```python
from build123d import *

# Parameters (mm, degrees)
F1_DEPTH = 14
F3_DEPTH = 23.7
F4_R     = 2


with BuildPart() as f1:
    # F0 (on Front) → F1 (new body)
    with BuildSketch(Plane.XZ):
        with BuildLine():
            ThreePointArc((27, -8.005587), (26.611392, -6.072957), (25.505976, -4.440741))
            ThreePointArc((25.505976, -4.440741), (13.780093, 3.288774), (0, 6))
            ThreePointArc((0, 6), (-13.780093, 3.288774), (-25.505976, -4.440741))
            ThreePointArc((-25.505976, -4.440741), (-26.611392, -6.072957), (-27, -8.005587))
            Line((-27, -8.005587), (-27, -21))
            ThreePointArc((-27, -21), (-24.071068, -28.071068), (-17, -31))
            Line((-17, -31), (17, -31))
            ThreePointArc((17, -31), (24.071068, -28.071068), (27, -21))
            Line((27, -21), (27, -8.005587))
        make_face()
        with BuildLine():
            ThreePointArc((-22, -8.005587), (0, 1), (22, -8.005587))
            Line((22, -8.005587), (22, -21))
            ThreePointArc((22, -21), (20.535534, -24.535534), (17, -26))
            Line((17, -26), (-17, -26))
            ThreePointArc((-17, -26), (-20.535534, -24.535534), (-22, -21))
            Line((-22, -21), (-22, -8.005587))
        make_face(mode=Mode.SUBTRACT)
    extrude(amount=F1_DEPTH)

    # F2 (on Top) → F3 (cut)
    with BuildSketch(Plane.XY):
        with BuildLine():
            ThreePointArc((0, -8.25), (0.883883, -7.883883), (1.25, -7))
            ThreePointArc((1.25, -7), (0.883883, -6.116117), (0, -5.75))
            Line((0, -5.75), (0, -8.25))
        make_face()
        with BuildLine():
            Line((0, -8.25), (0, -5.75))
            ThreePointArc((0, -5.75), (-1.25, -7), (0, -8.25))
        make_face()
    extrude(amount=F3_DEPTH, mode=Mode.SUBTRACT)

    # F4
    f4_edges = [f1.edges().sort_by_distance(p)[0] for p in [
        (0, -14, 1),
        (22, -14, -14.502794),
        (20.535534, -14, -24.535534),
        (0, 0, -26),
        (0, 0, 1),
        (0, 0, -31),
        (0, -14, -31),
    ]]
    fillet(f4_edges, radius=F4_R)


solid = f1.part
```
CAD build for the part. Positions are in the model's coordinates, mm. A direction names the side the tool comes from. Round coordinates to 2 decimals unless told otherwise and drop trailing zeros. Loops run counter-clockwise (first coordinate to the right, second up) from the corner with the lowest first, then second, coordinate; pieces in that order, holes last. Notation, with made-up numbers: M 83.25,40 L 91.25,40 A22 cw 91.25,72 Z; hole C 52,-17 d10. An arc over 180 degrees is marked long. Use a Markdown table: item, result. Add a question column.
(1) Cut at A-A (z = -19). Give the cut face in (x, y), and give its area (3 significant figures).
(2) Which spindle directions (+Z, -Z, +X, -X, +Y, -Y) get a long thin tool onto all of the face, cutting with end or side? Do faces 1 (the face through (-0.24, -0.57, -26.6)), 2 (the face through (-22.6, -13.43, -13.99)), 3 (the face through (0, -5, 1)), 4 (the face through (-27, -7, -14)), 5 (the face through (-24.15, -6.93, -27.99)). Say none if no direction does.
(3) Pull direction X, two halves, no side cores. Call faces 6 (the face through (-26.4, -13.43, -14.59)), 7 (the face through (22.6, -0.57, -14.19)), 8 (the face through (-3.8, 0, -28.3)): +X half, -X half, draft (parallel to the pull), parting line (faces both ways), or undercut.
(4) Cut at B-B (y = -3.75). Give the cut face in (x, z) (3 decimals), and give its area (3 significant figures).
(5) Cut at C-C (y = -1). Give the cut face in (x, z) (3 decimals), and give its area (3 significant figures).
(6) Drill centre lines: line 1 (X direction, y = -2.5, z = -13); line 2 (Z direction, x = -1, y = -5.25); line 3 (Z direction, x = 20, y = -0.5). Where is each one in solid material? Low to high.
(7) Flat gauge pins, fed straight in: pin 1 (1 mm diameter, centred on y = -7, z = -25, fed in from -X); pin 2 (1.5 mm diameter, centred on x = 13, y = -4, fed in from +Z); pin 3 (10 mm diameter, centred on x = 8, z = -18.5, fed in from -Y); pin 4 (2 mm diameter, centred on x = 6, y = -3, fed in from +Z). Where does each tip first touch, or does it go through?
Geometry says:
| question | item | result |
|---|---|---|
| 1 | outline | M -27,-12 A2 ccw -25,-14 L -24,-14 A2 ccw -22,-12 L -22,-2 A2 ccw -24,0 L -25,0 A2 ccw -27,-2 Z; M 22,-12 A2 ccw 24,-14 L 25,-14 A2 ccw 27,-12 L 27,-2 A2 ccw 25,0 L 24,0 A2 ccw 22,-2 Z |
| 1 | area | 133 mm² |
| 2 | face 1 | +Y |
| 2 | face 2 | -Y |
| 2 | face 3 | +Y, -Y |
| 2 | face 4 | +Z, -Z, -X, +Y, -Y |
| 2 | face 5 | -Z, -X, +Y, -Y |
| 3 | face 6 | -X half |
| 3 | face 7 | undercut |
| 3 | face 8 | draft |
| 4 | outline | M -27,-21 A10 ccw -17,-31 L 17,-31 A10 ccw 27,-21 L 27,-8.006 A5 ccw 25.506,-4.441 A36.375 ccw 0,6 A36.375 ccw -25.506,-4.441 A5 ccw -27,-8.006 Z; hole M -22,-21 A5 ccw -17,-26 L 17,-26 A5 ccw 22,-21 L 22,-8.006 A31.375 ccw -22,-8.006 Z |
| 4 | area | 701 mm² |
| 5 | outline | M -26.732,-21 A9.732 ccw -17,-30.732 L 17,-30.732 A9.732 ccw 26.732,-21 L 26.732,-8.006 A4.732 ccw 25.318,-4.632 A36.107 ccw 0,5.732 A36.107 ccw -25.318,-4.632 A4.732 ccw -26.732,-8.006 Z; hole M -22.268,-21 A5.268 ccw -17,-26.268 L 17,-26.268 A5.268 ccw 22.268,-21 L 22.268,-7.894 A31.643 ccw -22.268,-7.894 Z |
| 5 | area | 626 mm² |
| 6 | line 1 | x = -27 to -22, 22 to 27 |
| 6 | line 2 | z = -31 to -26, 0.98 to 5.99 |
| 6 | line 3 | z = -29.83 to -25.82, -5.33 to -0.81 |
| 7 | pin 1 | stops at x = -26.37 |
| 7 | pin 2 | stops at z = 3.88 |
| 7 | pin 3 | passes through |
| 7 | pin 4 | stops at z = 5.65 |
